from build123d import *

# Parameters (mm, degrees)
BOSS_EXTRUDE1_DEPTH = 3.96
SKETCH3_R           = 7.655
SKETCH3_R_2         = 1.75
SKETCH3_R_3         = 1.5
CUT_EXTRUDE1_DEPTH  = 50.655630094
FILLET2_R           = 7.025


with BuildPart() as part:
    # Sketch1 → Boss-Extrude1 (new body)
    with BuildSketch(Plane(origin=(0, 0, 0), x_dir=(1, 0, 0), z_dir=(0, 1, 0))):
        Polygon((35, 7.025), (7.025, 7.025), (7.025, 35), (-7.025, 35), (-7.025, 7.025), (-35, 7.025), (-35, -7.025), (-7.025, -7.025), (-7.025, -35), (7.025, -35), (7.025, -7.025), (35, -7.025), align=None)
    extrude(amount=BOSS_EXTRUDE1_DEPTH)

    # Sketch3 → Cut-Extrude1 (cut, through all)
    with BuildSketch(Plane(origin=(0, 0, 0), x_dir=(1, 0, 0), z_dir=(0, 1, 0))):
        with Locations(Location((0, 0, 0), (0, 0, 270))):
            Circle(SKETCH3_R)
        with Locations(Location((-14.88, 0, 0), (0, 0, 270))):
            Circle(SKETCH3_R_2)
        with Locations(Location((-28, 0, 0), (0, 0, 270))):
            Circle(SKETCH3_R_3)
        with Locations(Location((28, 0, 0), (0, 0, 90))):
            Circle(SKETCH3_R_3)
        with Locations(Location((14.88, 0, 0), (0, 0, 90))):
            Circle(SKETCH3_R_2)
        with Locations(Location((0, 14.88, 0), (0, 0, 270))):
            Circle(SKETCH3_R_2)
        with Locations(Location((0, 28, 0), (0, 0, 270))):
            Circle(SKETCH3_R_3)
        with Locations(Location((0, -28, 0), (0, 0, 90))):
            Circle(SKETCH3_R_3)
        with Locations(Location((0, -14.88, 0), (0, 0, 90))):
            Circle(SKETCH3_R_2)
    extrude(amount=CUT_EXTRUDE1_DEPTH, mode=Mode.SUBTRACT)

    # Fillet2
    fillet2_edges = [part.edges().sort_by_distance(p)[0] for p in [
        (7.025, 1.98, 7.025),
        (7.025, 1.98, -7.025),
        (-7.025, 1.98, -7.025),
        (-7.025, 1.98, 7.025),
        (35, 1.98, -7.025),
        (35, 1.98, 7.025),
        (7.025, 1.98, 35),
        (-7.025, 1.98, 35),
        (-35, 1.98, 7.025),
        (-35, 1.98, -7.025),
        (7.025, 1.98, -35),
        (-7.025, 1.98, -35),
    ]]
    fillet(fillet2_edges, radius=FILLET2_R - 0.0001)  # a hair under: the kernel refuses the full size


solid = part.part
Work out the finished part from the listing and answer in its coordinate system (mm). A direction names the side the tool comes from. Coordinates: 2 decimals unless noted, no trailing zeros. Loops run counter-clockwise (first coordinate to the right, second up) from the corner with the lowest first, then second, coordinate; pieces in that order, holes last. Notation, with made-up numbers: (30.5, -31) -> (73.5, -31) arc R14 ccw to (73.5, -12) -> close; hole circle Ø5 at (67, 74.25). An arc over 180 degrees is marked (long way). Answer as CSV lines item,"result".
1) The part is cut by section B-B (x = -6). Give the vertices of the cut face in (y, z).
A:
outline,"(0, -31.63) -> (3.96, -31.63) -> (3.96, -4.75) -> (0, -4.75) -> close; (0, 4.75) -> (3.96, 4.75) -> (3.96, 31.63) -> (0, 31.63) -> close"
2) Flat-ended cylindrical pins translate along their axes: pin 1 (1.5 mm diameter, centred on x = 11, y = 3.5, fed in from +Z); pin 2 (2.5 mm diameter, centred on x = -28, z = 0, fed in from -Y); pin 3 (1.5 mm diameter, centred on y = 3, z = 3.5, fed in from -X); pin 4 (2 mm diameter, centred on y = 2, z = 20, fed in from -X) (3 decimals). Find the tip coordinate at first contact, or state that the pin passes through.
A:
pin 1,"stops at z = 8.14"
pin 2,"passes through"
pin 3,"stops at x = -34.44"
pin 4,"stops at x = -7.025"
3) Straight lines are drawn through the part: probe 1 along X at (y, z) = (2.2, 0) (3 decimals); probe 2 along Z at (x, y) = (-28, 1.6); probe 3 along X at (y, z) = (2.65, 14.88) (3 decimals). For each, find the intervals that lie inside material, in ascending order.
A:
probe 1,"x = -35 to -29.5, -26.5 to -16.63, -13.13 to -7.655, 7.655 to 13.13, 16.63 to 26.5, 29.5 to 35"
probe 2,"z = -7.02 to -1.5, 1.5 to 7.02"
probe 3,"x = -7.025 to -1.75, 1.75 to 7.025"
4) The part is cut by section A-A (z = -14.88). Give the vertices of the cut face in (x, y) (3 decimals), and give its area (3 significant figures).
A:
outline,"(-7.025, 0) -> (-1.75, 0) -> (-1.75, 3.96) -> (-7.025, 3.96) -> close; (1.75, 0) -> (7.025, 0) -> (7.025, 3.96) -> (1.75, 3.96) -> close"
area,"41.8 mm²"
5) For faces 4 (the face through (-7.025, 2, 21)), 5 (the face through (0.526, 1.952, -13.211)), 6 (the face through (21, 2, -7.025)), 7 (the face through (-21, 2, -7.025)), determine the directions among +Z, -Z, +X, -X, +Y, -Y from which every point of the face is accessible in a straight line to the end or side of a thin tool.
A:
face 4,"+Z, -X, +Y, -Y"
face 5,"+Y, -Y"
face 6,"-Z, +X, +Y, -Y"
face 7,"-Z, -X, +Y, -Y"
6) The part is cut by section C-C (y = 2.1). State how many separate pieces and enclosed holes the cut face has, and give its area (3 significant figures).
A:
separate pieces,"1"
enclosed holes,"9"
area,"1,480 mm²"
7) The part is cut by section D-D (x = -21). Give the vertices of the cut face in (y, z) (3 decimals).
A:
outline,"(0, -7.025) -> (3.96, -7.025) -> (3.96, 7.025) -> (0, 7.025) -> close"
8) For a pull along Z with two mould halves and no side action, classify faces 1 (the face through (7.025, 2, 21)), 2 (the face through (-9.028, 2.008, -9.137)), 3 (the face through (7.59, 1.95, -1)) as released by +Z, released by -Z, zero draft, split by the parting line, or undercut.
A:
face 1,"zero draft"
face 2,"released by -Z"
face 3,"undercut"
